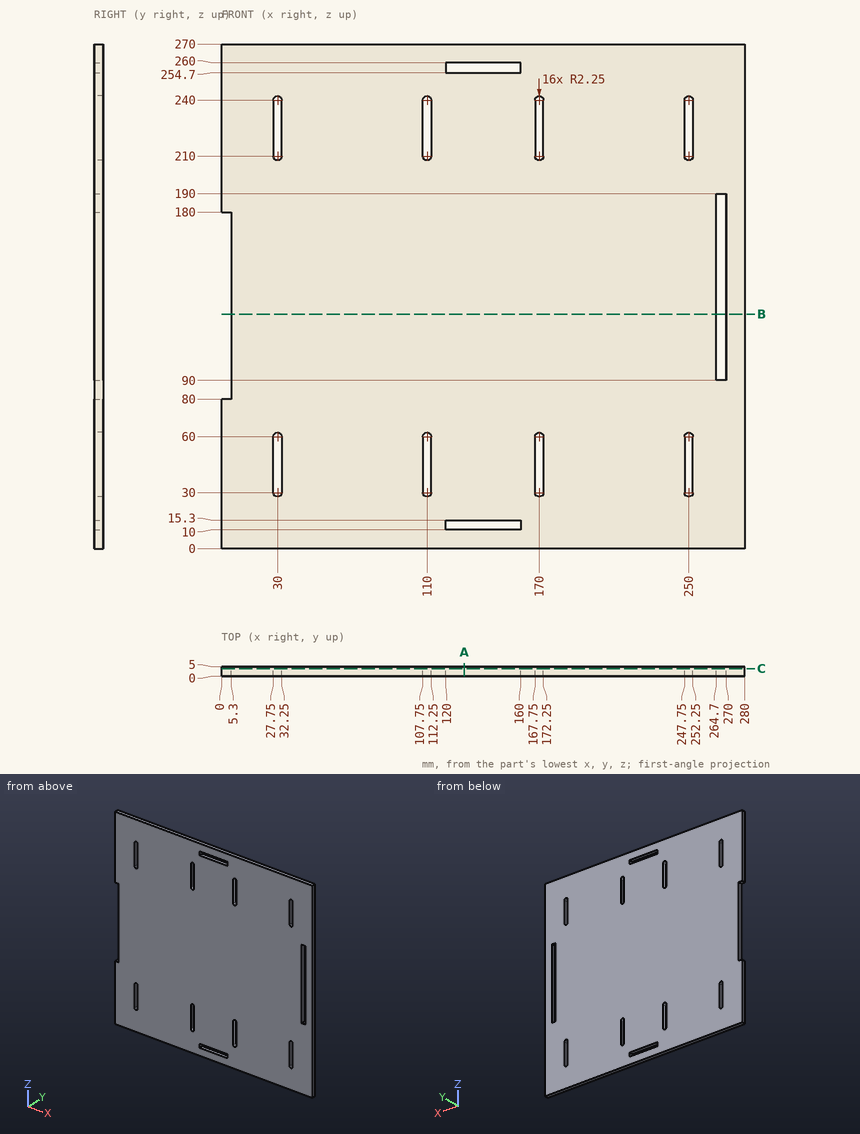
Job drawing, mm, ordinate dimensions from the low corner. One solid piece. Coordinates: 2 decimals unless noted, no trailing zeros. Order: outer loops, then holes, each group sorted by start corner. A loop starts at its lowest first (then second) coordinate and runs counter-clockwise, first axis right, second up. Notation, with made-up numbers: M 44.25,42 L 77.25,42 A12 ccw 77.25,46 Z; hole C -6,-23.75 d3. An arc over 180 degrees is marked long. Answer as CSV lines item,"result".
(1) Band-saw the part on B-B, the plane z = 125.5. List the corners of the cut face in (x, y).
Geometry says:
outline,"M 5.3,0 L 264.7,0 L 264.7,5 L 5.3,5 Z; M 270,0 L 280,0 L 280,5 L 270,5 Z"
(2) Wall check: line 1 along Z through (x, y) = (150.5, 2.45); line 2 along X through (y, z) = (3.8, 213); line 3 along X through (y, z) = (3.55, 166). Give the ranges that are in metal, low to high.
Geometry says:
line 1,"z = 0 to 10, 15.3 to 254.7, 260 to 270"
line 2,"x = 0 to 27.75, 32.25 to 107.75, 112.25 to 167.75, 172.25 to 247.75, 252.25 to 280"
line 3,"x = 5.3 to 264.7, 270 to 280"
(3) Band-saw the part on C-C, the plane y = 3.9. State how many separate pieces and enclosed holes the cut face has, then the cut area to 3 significant figures.
Geometry says:
separate pieces,"1"
enclosed holes,"11"
area,"72,900 mm2"
(4) Band-saw the part on A-A, the plane x = 130. List the corners of the cut face in (y, z), then the cut area to 3 significant figures.
Geometry says:
outline,"M 0,0 L 5,0 L 5,10 L 0,10 Z; M 0,15.3 L 5,15.3 L 5,254.7 L 0,254.7 Z; M 0,260 L 5,260 L 5,270 L 0,270 Z"
area,"1,300 mm2"
